Autodesk Inventor part; units mm, degrees
ref_plane "YZ Plane" through (0, 0, 0) normal (1, 0, 0) x (0, 1, 0)
ref_plane "XZ Plane" through (0, 0, 0) normal (0, 1, 0) x (-1, 0, 0)
ref_plane "XY Plane" through (0, 0, 0) normal (0, 0, 1) x (1, 0, 0)
sketch "Sketch1" plane through (0, 0, 0) normal (0, 0, 1) x (1, 0, 0)
  line L0 (6.1879, 20.8703) -> (36.1879, 20.8703)
  line L1 (36.1879, -14.1297) -> (6.1879, -14.1297)
  line L2 (39.1879, 23.8703) -> (3.1879, 23.8703)
  line L3 (3.1879, -17.1297) -> (39.1879, -17.1297)
  line L4 (56.1879, 23.8703) -> (59.1879, 23.8703)
  line L5 (59.1879, 23.8703) -> (59.1879, -17.1297)
  line L6 (59.1879, -17.1297) -> (39.1879, -17.1297)
  line L7 (56.1879, 20.8703) -> (56.1879, -14.1297)
  line L8 (56.1879, -14.1297) -> (39.1879, -14.1297)
  line L9 (36.1879, 20.8703) -> (36.1879, 13.8703)
  line L10 (36.1879, 13.8703) -> (39.1879, 13.8703)
  line L11 (36.1879, -14.1297) -> (36.1879, -7.1297)
  line L12 (36.1879, -7.1297) -> (39.1879, -7.1297)
  line L13 (36.1879, 20.8703) -> (36.1879, 13.8703)
  line L14 (36.1879, -7.1297) -> (36.1879, -14.1297)
  line L15 (39.1879, -14.1297) -> (39.1879, -7.1297)
  line L16 (39.1879, 13.8703) -> (39.1879, 20.8703)
  line L17 (3.1879, 23.8703) -> (3.1879, 20.8703)
  line L18 (3.1879, -14.1297) -> (3.1879, -17.1297)
  line L19 (6.1879, 20.8703) -> (3.1879, 20.8703)
  line L20 (6.1879, -14.1297) -> (3.1879, -14.1297)
  line L21 (39.1879, 20.8703) -> (39.1879, 23.8703)
  line L22 (56.1879, 20.8703) -> (56.1879, 23.8703)
  point P0 (0, 0)
  dimension "d1" = 35
  dimension "d2" = 3
  dimension "d3" = 20
  dimension "d5" = 7
  dimension "d6" = 7
  dimension "d7" = 30
extrude "Extrusion1" add sketch "Sketch1" along normal mid plane 35
sketch "Sketch2" plane through (0, 0, -17.5) normal (0, 0, -1) x (-1, 0, 0)
  line L0 (-59.1879, 23.8703) -> (-3.1879, 23.8703)
  line L1 (-3.1879, -17.1297) -> (-59.1879, -17.1297)
  line L2 (-59.1879, 23.8703) -> (-3.1879, 23.8703)
  line L3 (-3.1879, 23.8703) -> (-3.1879, -17.1297)
  line L4 (-3.1879, -17.1297) -> (-59.1879, -17.1297)
  line L5 (-59.1879, -17.1297) -> (-59.1879, 23.8703)
  point P0 (0, 0)
extrude "Extrusion3" add sketch "Sketch2" along normal blind 3
sketch "Sketch3" plane through (0, 0, 17.5) normal (0, 0, 1) x (1, 0, 0)
  line L0 (3.1879, 23.8703) -> (59.1879, 23.8703)
  line L1 (59.1879, -17.1297) -> (3.1879, -17.1297)
  line L2 (3.1879, 23.8703) -> (59.1879, 23.8703)
  line L3 (59.1879, 23.8703) -> (59.1879, -17.1297)
  line L4 (59.1879, -17.1297) -> (3.1879, -17.1297)
  line L5 (3.1879, -17.1297) -> (3.1879, 23.8703)
  point P0 (0, 0)
extrude "Extrusion4" add sketch "Sketch3" along normal blind 3
sketch "Sketch4" plane through (3.1879, -14.1297, -17.5) normal (0, 1, 0) x (1, 0, 0)
  line L0 (56, 3) -> (0, 3)
  line L1 (0, 3) -> (56, 3)
  line L2 (0, -38) -> (56, -38)
  line L3 (56, 3) -> (56, -38)
  line L4 (33, 0) -> (33, -35)
  circle A0 centre (33, -17.5) radius 4
  point P0 (-3.1879, -17.5)
  dimension "d18" = 8
extrude "Extrusion5" cut sketch "Sketch4" along normal mid plane 15
Here's how the part is built. I have some questions about the finished solid (model axes, mm). A direction names the side the tool comes from. Coordinates: 2 decimals unless noted, no trailing zeros. Loops run counter-clockwise (first coordinate to the right, second up) from the corner with the lowest first, then second, coordinate; pieces in that order, holes last. Notation, with made-up numbers: (60, 75) -> (110, 75) arc R15 cw to (110, 84) -> close; hole circle Ø3 at (-33, -26.75). An arc over 180 degrees is marked (long way). Return JSON: item names as keys, results as strings.
1) If we section it at A-A, the plane z = -12: Write out the boundary of the cut face in (x, y), then the cut area to 3 significant figures.
Results below:
{"outline": "(3.19, -17.13) -> (59.19, -17.13) -> (59.19, 23.87) -> (56.19, 23.87) -> (56.19, -14.13) -> (39.19, -14.13) -> (39.19, -7.13) -> (36.19, -7.13) -> (36.19, -14.13) -> (3.19, -14.13) -> close; (3.19, 20.87) -> (36.19, 20.87) -> (36.19, 13.87) -> (39.19, 13.87) -> (39.19, 23.87) -> (3.19, 23.87) -> close", "area": "432 mm²"}
2) For faces 1 (the face through (39.188, -11, 10)), 2 (the face through (32, -17.13, 0)), 3 (the face through (40.003, -14.282, -1.201)), 4 (the face through (38, -7.13, -10)), 5 (the face through (30, 5, -17.5)), which set-ups out of +Z, -Z, +X, -X, +Y, -Y let a thin tool reach every point of the face, with its end or its side?
Results below:
{"face 1": "+Y", "face 2": "+Z, -Z, +X, -X, -Y", "face 3": "-Y", "face 4": "-X", "face 5": "none"}
3) I need wall thicknesses on line 1 (Y direction, x = 13, z = 9); line 2 (X direction, y = -15, z = 0); line 3 (Z direction, x = 14.5, y = -5). Which ranges of each line are inside material? Lowest first, please. Write a range as from..to.
Results below:
{"line 1": "-17.13..-14.13, 20.87..23.87", "line 2": "3.19..32.19, 40.19..59.19", "line 3": "-20.5..-17.5, 17.5..20.5"}
4) If we section it at B-B, the plane x = 50.5: Write out the boundary of the cut face in (y, z), then the cut area to 3 significant figures.
Results below:
{"outline": "(-17.13, -20.5) -> (23.87, -20.5) -> (23.87, -17.5) -> (-14.13, -17.5) -> (-14.13, 17.5) -> (23.87, 17.5) -> (23.87, 20.5) -> (-17.13, 20.5) -> close", "area": "351 mm²"}
5) Thinking about a two-plate mould opening in Y: for faces 6 (the face through (48, -14.13, 0)), 7 (the face through (20, -14.13, 0)), 8 (the face through (39.188, -11, -10)), 9 (the face through (38, 13.87, 0)), which applies, +Y half, -Y half, draft (parallel to the pull), parting line (faces both ways), or undercut?
Results below:
{"face 6": "+Y half", "face 7": "undercut", "face 8": "draft", "face 9": "undercut"}
6) If we section it at D-D, the plane y = -8: Write out the boundary of the cut face in (x, z).
Results below:
{"outline": "(3.19, -20.5) -> (59.19, -20.5) -> (59.19, 20.5) -> (3.19, 20.5) -> (3.19, 17.5) -> (36.19, 17.5) -> (36.19, 4) arc R4 cw to (39.19, 2.65) -> (39.19, 17.5) -> (56.19, 17.5) -> (56.19, -17.5) -> (39.19, -17.5) -> (39.19, -2.65) arc R4 cw to (36.19, -4) -> (36.19, -17.5) -> (3.19, -17.5) -> close"}
7) Will these pins go through, and if not, where does the flat tip stop? pin 1 (5 mm diameter, centred on x = 45.5, z = -8.5, fed in from +Y); pin 2 (7.5 mm diameter, centred on y = -9.5, z = -13, fed in from -X).
Results below:
{"pin 1": "y = -14.13", "pin 2": "x = 36.19"}
8) If we section it at C-C, the plane z = 0: Write out the boundary of the cut face in (x, y).
Results below:
{"outline": "(3.19, -17.13) -> (32.19, -17.13) -> (32.19, -14.13) -> (3.19, -14.13) -> close; (3.19, 20.87) -> (36.19, 20.87) -> (36.19, 13.87) -> (39.19, 13.87) -> (39.19, 23.87) -> (3.19, 23.87) -> close; (40.19, -17.13) -> (59.19, -17.13) -> (59.19, 23.87) -> (56.19, 23.87) -> (56.19, -14.13) -> (40.19, -14.13) -> close"}
